Here's how the part is built. I have some questions about the finished solid (model axes, mm). A direction names the side the tool comes from. Round coordinates to 2 decimals unless told otherwise and drop trailing zeros. Order: outer loops, then holes, each group sorted by start corner. A loop starts at its lowest first (then second) coordinate and runs counter-clockwise, first axis right, second up. Notation, with made-up numbers: M 74,68 L 100,68 A21 ccw 100,80 Z; hole C 3.5,34 d9. An arc over 180 degrees is marked long. Write item = value, one per line. Start each with the question number.
Item 1: We'd pull the mould along X, two halves only. Please class faces 1 (the face through (10.9, 1, 8.8)), 2 (the face through (0, -20, -9)), 3 (the face through (17.5, -4.1, -8.2)): pulls with the +X half, pulls with the -X half, needs draft (parallel to the pull), parting line crosses it, or undercut.
Item 2: I want a section at B-B, the plane x = 2. List the corners of the cut face in (y, z) for me, plus the area to 3 significant figures.
Item 3: I'm going to push flat-ended pins straight in: P1, Ø3, axis at x = -11.5, z = 8, coming from the -Y side; P2, Ø10, axis at x = -9, y = -9, coming from the +Z side. Where does each tip first touch, or does it pass through?
Item 4: I want a section at D-D, the plane z = 8. List the corners of the cut face in (x, y) for me, plus the area to 3 significant figures.
Item 5: I want a section at C-C, the plane y = -8. List the corners of the cut face in (x, z) for me.
Item 6: I want a section at A-A, the plane z = 2.5. List the corners of the cut face in (x, y) for me, plus the area to 3 significant figures.
Item 7: For faces 4 (the face through (0, 0, -3)), 5 (the face through (-17.5, -4.1, -8.2)), which set-ups out of +Z, -Z, +X, -X, +Y, -Y let a thin tool reach every point of the face, with its end or its side?
Item 8: Please list where these lines run through material, in increasing order: L1, parallel to X at y = 0.5, z = 8; L2, parallel to Y at x = 4.5, z = 7.25; L3, parallel to Z at x = -12, y = -6.5.
```python
from build123d import *

# Parameters (mm, degrees)
SKETCH1_W           = 35
SKETCH1_H           = 20
BOSS_EXTRUDE1_DEPTH = 2
SKETCH2_W           = 35
SKETCH2_H           = 2
BOSS_EXTRUDE2_DEPTH = 20
SKETCH3_R           = 1.5
CUT_EXTRUDE1_DEPTH  = 20
SKETCH4_R           = 1
CUT_EXTRUDE2_DEPTH  = 20
SKETCH6_R           = 2.5
CUT_EXTRUDE3_DEPTH  = 20


with BuildPart() as part:
    # Sketch1 → Boss-Extrude1 (new body)
    with BuildSketch(Plane(origin=(0, 0, 0), x_dir=(1, 0, 0), z_dir=(0, 1, 0))):
        Rectangle(SKETCH1_W, SKETCH1_H)
    extrude(amount=BOSS_EXTRUDE1_DEPTH)

    # Sketch2 → Boss-Extrude2 (add)
    with BuildSketch(Plane.XZ):
        with Locations((0, -9)):
            Rectangle(SKETCH2_W, SKETCH2_H)
    extrude(amount=BOSS_EXTRUDE2_DEPTH)

    # Sketch3 → Cut-Extrude1 (cut)
    with BuildSketch(Plane(origin=(0, 0, -10), x_dir=(-1, 0, 0), z_dir=(0, 0, -1))):
        with Locations((-15.240565198, -8)):
            Circle(SKETCH3_R)
        with Locations((15.443232288, -8)):
            Circle(SKETCH3_R)
    extrude(amount=-CUT_EXTRUDE1_DEPTH, mode=Mode.SUBTRACT)

    # Sketch4 → Cut-Extrude2 (cut)
    with BuildSketch(Plane.XZ):
        with Locations(Location((-11.5, 8, 0), (0, 0, 270))):
            Circle(SKETCH4_R)
        with Locations(Location((11.5, 8, 0), (0, 0, 270))):
            Circle(SKETCH4_R)
    extrude(amount=-CUT_EXTRUDE2_DEPTH, mode=Mode.SUBTRACT)

    # Sketch6 → Cut-Extrude3 (cut)
    with BuildSketch(Plane.XZ):
        with Locations(Location((0, 1, 0), (0, 0, 270))):
            Circle(SKETCH6_R)
    extrude(amount=-CUT_EXTRUDE3_DEPTH, mode=Mode.SUBTRACT)


solid = part.part
```
Filled in:
q1.face_1 = undercut
q1.face_2 = needs draft
q1.face_3 = pulls with the +X half
q2.outline = M -20,-10 L 2,-10 L 2,-0.5 L 0,-0.5 L 0,-8 L -20,-8 Z; M 0,2.5 L 2,2.5 L 2,10 L 0,10 Z
q2.area = 74.0 mm^2
q3.P1 = 0
q3.P2 = -8
q4.outline = M -17.5,0 L -12.5,0 L -12.5,2 L -17.5,2 Z; M -10.5,0 L 10.5,0 L 10.5,2 L -10.5,2 Z; M 12.5,0 L 17.5,0 L 17.5,2 L 12.5,2 Z
q4.area = 62.0 mm^2
q5.outline = M -17.5,-10 L -16.94,-10 L -16.94,-8 L -17.5,-8 Z; M -13.94,-10 L 13.74,-10 L 13.74,-8 L -13.94,-8 Z; M 16.74,-10 L 17.5,-10 L 17.5,-8 L 16.74,-8 Z
q6.outline = M -17.5,0 L -2,0 L -2,2 L -17.5,2 Z; M 2,0 L 17.5,0 L 17.5,2 L 2,2 Z
q6.area = 62.0 mm^2
q7.face_4 = +Z, +X, -X, -Y
q7.face_5 = +Z, -Z, -X, +Y, -Y
q8.L1 = -17.5 to -12.5, -10.5 to 10.5, 12.5 to 17.5
q8.L2 = 0 to 2
q8.L3 = -10 to -8
